Geometry check sheet. Reference: the model listing, model coordinates, mm. Face numbers are marked on the shaded views. Round coordinates to 2 decimals unless told otherwise and drop trailing zeros. Order: outer loops, then holes, each group sorted by start corner. A loop starts at its lowest first (then second) coordinate and runs counter-clockwise, first axis right, second up. Notation, with made-up numbers: (31.5, 89.5) -> (69.5, 89.5) arc R17 ccw to (69.5, 122.5) -> close; hole circle Ø5 at (-4, -26). An arc over 180 degrees is marked (long way). Use a Markdown table: item, result. Add a question column.
Item 1: Gauge pin test, flat ends, axial feed: pin 1 Ø1 at (x, z) = (-1, 1.5) entering from +Y; pin 2 Ø1 at (y, z) = (2.5, 6) entering from -X; pin 3 Ø8 at (x, y) = (14.5, -10.5) entering from -Z; pin 4 Ø1 at (x, y) = (-0.5, 0.5) entering from +Z. Record the tip position at first contact, or that the pin passes through.
Item 2: Material ranges on probe 1 along Y at (x, z) = (13, 1); probe 2 along X at (y, z) = (-12.5, 1); probe 3 along Z at (x, y) = (2, 4.5), recorded low to high. Write a range as [from, to].
Item 3: Sectioned sample at D-D, the plane y = -11. Record the cut outline in (x, z).
Item 4: Sectioned sample at B-B, the plane y = 4. Record the cut outline in (x, z), and give its area (3 significant figures).
Item 5: Mould release check, pull along X, two halves, no side actions. Record for the marked faces 1 and 2: pulls with the +X half, pulls with the -X half, needs draft (parallel to the pull), parting line crosses it, or undercut.
Item 6: Sectioned sample at A-A, the plane x = -10.5. Record the cut outline in (y, z), and give its area (3 significant figures).
Item 7: Sectioned sample at C-C, the plane z = 6. Record the cut outline in (x, y), and give its area (3 significant figures).
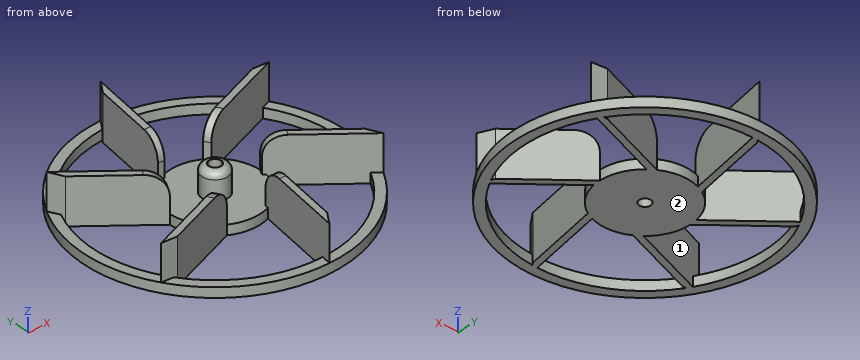
from build123d import *

# Parameters (mm, degrees)
SKETCH_R           = 7
PAD_DEPTH          = 1.5
PAD001_DEPTH       = 7
POLARPATTERN_COUNT = 6
SKETCH002_R        = 20
SKETCH002_R_2      = 18.52462
PAD002_DEPTH       = 1.5
SKETCH003_R        = 2
PAD003_DEPTH       = 4
SKETCH004_R        = 0.9
POCKET_DEPTH       = 10
FILLET_R           = 1
FILLET001_R        = 3


with BuildPart() as part:
    # Sketch → Pad (new body)
    with BuildSketch(Plane.XY):
        Circle(SKETCH_R)
    extrude(amount=PAD_DEPTH)

    # Sketch001 → Pad001 (new body)
    with BuildSketch(Plane(origin=(0, 0, 0), x_dir=(1, 0, 0), z_dir=(0, 0, -1))):
        Polygon((2.454578, 6.079397), (0, 20), (1.357197, 18.061721), (3.470004, 6.079397), align=None)
    pad001 = extrude(amount=-PAD001_DEPTH)

    # PolarPattern: Pad001 ×6 about axis
    polarpattern_axis = Axis((0, 0, 0), (0, 0, -1))
    for i in range(1, POLARPATTERN_COUNT):
        add(pad001.rotate(polarpattern_axis, i * 360 / POLARPATTERN_COUNT))

    # Sketch002 → Pad002 (new body)
    with BuildSketch(Plane(origin=(0, 0, 0), x_dir=(1, 0, 0), z_dir=(0, 0, -1))):
        Circle(SKETCH002_R)
        Circle(SKETCH002_R_2, mode=Mode.SUBTRACT)
    extrude(amount=-PAD002_DEPTH)

    # Sketch003 → Pad003 (new body)
    with BuildSketch(Plane.XY.offset(1.5)):
        Circle(SKETCH003_R)
    extrude(amount=PAD003_DEPTH)

    # Sketch004 → Pocket (cut)
    with BuildSketch(Plane.XY.offset(5.5)):
        Circle(SKETCH004_R)
    extrude(amount=-POCKET_DEPTH, mode=Mode.SUBTRACT)

    # Fillet
    fillet_edges = [part.edges().sort_by_distance(p)[0] for p in [
        (-2, 0, 5.5),
    ]]
    fillet(fillet_edges, radius=FILLET_R)

    # Fillet001
    fillet001_edges = [part.edges().sort_by_distance(p)[0] for p in [
        (2.962291, -6.079397, 7),
        (-3.783767, -5.605118, 7),
        (-6.746058, 0.474279, 7),
        (-2.962291, 6.079397, 7),
        (3.783767, 5.605118, 7),
        (6.746058, -0.474279, 7),
    ]]
    fillet(fillet001_edges, radius=FILLET001_R)


solid = part.part
Found:
| question | item | result |
|---|---|---|
| 1 | pin 1 | stops at y = 19.99 |
| 1 | pin 2 | stops at x = -10.53 |
| 1 | pin 3 | stops at z = 0 |
| 1 | pin 4 | stops at z = 5.5 |
| 2 | probe 1 | y = [-15.2, -13.2], [-6.37, -5.07], [8.43, 9.49], [13.2, 15.2] |
| 2 | probe 2 | x = [-15.61, -13.67], [1.32, 2.34], [13.67, 15.61] |
| 2 | probe 3 | z = [0, 1.5] |
| 3 | outline | (-16.7, 0) -> (-14.91, 0) -> (-14.91, 1.5) -> (-16.7, 1.5) -> close; (1.59, 0) -> (2.6, 0) -> (2.6, 7) -> (1.59, 7) -> close; (14.91, 0) -> (16.7, 0) -> (16.7, 1.5) -> (14.91, 1.5) -> close |
| 4 | outline | (-19.6, 0) -> (-18.09, 0) -> (-18.09, 1.5) -> (-19.6, 1.5) -> close; (-11.73, 0) -> (-10.17, 0) -> (-10.17, 7) -> (-11.73, 7) -> close; (-5.74, 0) -> (5.74, 0) -> (5.74, 1.5) -> (-5.74, 1.5) -> close; (18.09, 0) -> (19.6, 0) -> (19.6, 1.5) -> (18.09, 1.5) -> close |
| 4 | area | 32.6 mm2 |
| 5 | face 1 | undercut |
| 5 | face 2 | needs draft |
| 6 | outline | (-17.02, 0) -> (-15.26, 0) -> (-15.26, 1.5) -> (-17.02, 1.5) -> close; (-8.58, 0) -> (-7.52, 0) -> (-7.52, 7) -> (-8.58, 7) -> close; (2.97, 0) -> (4.28, 0) -> (4.28, 7) -> (2.97, 7) -> close; (15.26, 0) -> (17.02, 0) -> (17.02, 1.5) -> (15.26, 1.5) -> close |
| 6 | area | 21.9 mm2 |
| 7 | outline | (-17.32, -10) -> (-14.96, -10.21) -> (-4.26, -6.31) -> (-4.77, -5.43) -> close; (-17.32, 10) -> (-16.32, 7.86) -> (-7.59, 0.53) -> (-7.09, 1.41) -> close; (-3.34, 6.84) -> (-2.32, 6.84) -> (0, 20) -> (-1.36, 18.06) -> close; (0, -20) -> (1.36, -18.06) -> (3.34, -6.84) -> (2.32, -6.84) -> close; (4.26, 6.31) -> (4.77, 5.43) -> (17.32, 10) -> (14.96, 10.21) -> close; (7.09, -1.41) -> (17.32, -10) -> (16.32, -7.86) -> (7.59, -0.53) -> close |
| 7 | area | 74.3 mm2 |
